Model file for the job. Use its own axes, mm. A direction names the side the tool comes from. Round coordinates to 2 decimals unless told otherwise and drop trailing zeros. Order: outer loops, then holes, each group sorted by start corner. A loop starts at its lowest first (then second) coordinate and runs counter-clockwise, first axis right, second up. Notation, with made-up numbers: M -26,82.25 L 29,82.25 A23 ccw 29,116.25 Z; hole C 2,-23 d1. An arc over 180 degrees is marked long. Return JSON: item names as keys, results as strings. Group by question number.
Item 1: Pull direction Y, two halves, no side cores. Call faces 1 (the face through (129.029, 30.837, 0.74)), 2 (the face through (97, 36.65, 0.74)), 3 (the face through (130.937, 33.329, 0.74)): pulls with the +Y half, pulls with the -Y half, needs draft (parallel to the pull), parting line crosses it, or undercut.
Item 2: Probe line 1 along X through (y, z) = (44, 1.1); line 2 along Y through (x, z) = (36.5, 1.15); line 3 along Y through (x, z) = (79.5, 0.75). List the from-to ranges inside material, lowest first.
Item 3: Slice it at A-A on z = 0.25. Write the cut outline in (x, y).
Item 4: Slice it at B-B on y = 9. Write the cut outline in (x, z), then the cut area to 3 significant figures.
Item 5: Which spindle directions (+Z, -Z, +X, -X, +Y, -Y) get a long thin tool onto all of the face, cutting with end or side? Do faces 4 (the face through (36.141, 48.303, 0.74)), 5 (the face through (11.58, 53.26, 0.76)). Say none if no direction does.
Item 6: Slice it at C-C on x = 32. Write the cut outline in (y, z).
Autodesk Inventor part; units mm, degrees
ref_plane "YZ Plane" through (0, 0, 0) normal (1, 0, 0) x (0, 1, 0)
ref_plane "XZ Plane" through (0, 0, 0) normal (0, 1, 0) x (-1, 0, 0)
ref_plane "XY Plane" through (0, 0, 0) normal (0, 0, 1) x (1, 0, 0)
sketch "スケッチ1" plane through (0, 0, 0) normal (0, 0, 1) x (1, 0, 0)
  circle A0 centre (-35.9404, 22.842) radius 1.5
  circle A1 centre (5.9362, 53.5882) radius 1.5
  circle A2 centre (127.6431, 30.2622) radius 1.5
  line L0 (22.9895, 50.3198) -> (110.5899, 33.5306)
  circle A3 centre (5.9362, 53.5882) radius 4.5
  circle A4 centre (127.6431, 30.2622) radius 4.5
  circle A5 centre (-35.9404, 22.842) radius 3
  line L1 (5.0892, 49.1686) -> (9.9998, 48.2275)
  line L2 (9.9998, 48.2275) -> (22.9895, 50.3198)
  line L3 (110.5899, 33.5306) -> (121.8855, 26.7838)
  line L4 (121.8855, 26.7838) -> (126.7961, 25.8426)
  line L5 (4.4419, 57.8328) -> (15.2047, 61.622)
  line L6 (-37.785, 25.2079) -> (3.1694, 57.1371)
  line L7 (3.5126, 49.7966) -> (-34.0959, 20.4761)
  line L8 (122.0018, 41.1536) -> (130.601, 33.6535)
  circle A6 centre (80.3181, 36.2778) radius 3
  circle A7 centre (80.3181, 36.2778) radius 4.5
  line L9 (128.2106, 34.7263) -> (80.8855, 40.7419)
  circle A8 centre (80.4743, 23.124) radius 1.5
  line L10 (120.4636, 35.711) -> (121.0283, 38.6574)
  line L11 (15.1864, 58.9428) -> (14.6217, 55.9964)
  circle A9 centre (66.9779, 42.9073) radius 1.5
  circle A10 centre (66.9779, 42.9073) radius 3
  line L12 (29.9182, 56.1193) -> (29.3535, 53.1729)
  arc A11 (17.2488, 58.5475) -> (15.1864, 58.9428) centre (16.2176, 58.7451) ccw
  arc A12 (29.9182, 56.1193) -> (27.8558, 56.5146) centre (28.887, 56.3169) ccw
  arc A13 (27.2911, 53.5682) -> (29.3535, 53.1729) centre (28.3223, 53.3705) ccw
  arc A14 (14.6217, 55.9964) -> (16.6841, 55.6011) centre (15.6529, 55.7987) ccw
  line L13 (17.2488, 58.5475) -> (27.8558, 56.5146)
  line L14 (16.6841, 55.6011) -> (27.2911, 53.5682)
  arc A15 (31.8825, 55.7428) -> (27.0019, 58.7146) centre (28.887, 56.3169) ccw
  line L15 (27.0019, 58.7146) -> (18.8556, 60.2759)
  arc A16 (18.8556, 60.2759) -> (15.2047, 61.622) centre (16.2176, 58.7451) ccw
  line L16 (106.2964, 41.4808) -> (105.7317, 38.5345)
  arc A17 (108.3589, 41.0856) -> (106.2964, 41.4808) centre (107.3276, 41.2832) ccw
  arc A18 (121.0283, 38.6574) -> (118.9658, 39.0527) centre (119.997, 38.855) ccw
  arc A19 (118.4011, 36.1063) -> (120.4636, 35.711) centre (119.4323, 35.9086) ccw
  arc A20 (105.7317, 38.5345) -> (107.7942, 38.1392) centre (106.7629, 38.3368) ccw
  line L17 (31.8825, 55.7428) -> (104.3322, 41.8573)
  line L18 (108.3589, 41.0856) -> (118.9658, 39.0527)
  line L19 (107.7942, 38.1392) -> (118.4011, 36.1063)
  arc A21 (122.0018, 41.1536) -> (118.1119, 41.2527) centre (119.997, 38.855) ccw
  line L20 (118.1119, 41.2527) -> (109.9656, 42.814)
  arc A22 (109.9656, 42.814) -> (104.3322, 41.8573) centre (107.3276, 41.2832) ccw
  line L21 (30.451, 58.9354) -> (37.6452, 54.6383)
  line L22 (16.7917, 61.7406) -> (29.4611, 59.3124)
  line L23 (120.5711, 41.8505) -> (107.9017, 44.2787)
  line L24 (106.8426, 44.2944) -> (98.5694, 42.9618)
  point P0 (0, 0)
  point P1 (0, 0)
  dimension "d4" = 9
  dimension "d0" = 9
  dimension "d1" = 9
  dimension "d2" = 6
  dimension "d3" = 6
  dimension "d5" = 47.7059
  dimension "d6" = 47.7059
  dimension "d7" = 3
  dimension "d8" = 3
  dimension "d9" = 8.0769
  dimension "d10" = 8.0769
  dimension "d11" = 3
  dimension "d12" = 6
  dimension "d13" = 61.9691
  dimension "d14" = 61.9691
  dimension "d15" = 15
  dimension "d16" = 2.1
  dimension "d17" = 2
  dimension "d18" = 2
  dimension "d19" = 2
  dimension "d20" = 15
  dimension "d21" = 2.1
  dimension "d22" = 7
  dimension "d23" = 2
  dimension "d24" = 2
  dimension "d25" = 5
  dimension "d26" = 5
  dimension "d27" = 160
  dimension "d28" = 160
  dimension "d29" = 160
  dimension "d30" = 160
sketch "スケッチ2" plane through (0, 0, 0) normal (0, 0, 1) x (1, 0, 0)
  circle A0 centre (5.9362, 53.5882) radius 1.5
  circle A1 centre (66.9779, 42.9073) radius 1.5
  circle A2 centre (127.6431, 30.2622) radius 1.5
  arc A3 (10.3689, 52.8126) -> (1.6172, 52.3248) centre (5.9362, 53.5882) ccw
  arc A4 (71.3832, 41.9891) -> (62.5453, 43.6829) centre (66.9779, 42.9073) ccw
  arc A5 (130.338, 26.6583) -> (123.2378, 31.1804) centre (127.6431, 30.2622) ccw
  line L0 (10.3689, 52.8126) -> (62.5453, 43.6829)
  line L1 (71.3832, 41.9891) -> (123.2378, 31.1804)
  line L2 (130.338, 26.6583) -> (72.4655, -16.6159)
  line L3 (72.4655, -16.6159) -> (15.6298, 4.4202)
  line L4 (15.6298, 4.4202) -> (1.6172, 52.3248)
  point P0 (0, 0)
  dimension "d31" = 9
  dimension "d32" = 9
  dimension "d33" = 9
extrude "押し出し1" add sketch "スケッチ2" along normal blind 1.5
fillet "フィレット1" radius 5 4 edges at (10.3689, 52.8126, 0.75) (62.5453, 43.6829, 0.75) (71.3832, 41.9891, 0.75) (123.2378, 31.1804, 0.75)
equation "\"d6\" = d5"
equation "\"d10\" = d9"
equation "\"d14\" = d13"
properties part number "台形サスカバー" material "ポリカーボネート、クリア"
Output values:
{
 "1": {"face 1": "undercut", "face 2": "pulls with the +Y half", "face 3": "parting line crosses it"},
 "2": {"line 1": "4.05 to 65.95, 68.01 to 71.39", "line 2": "-3.3 to 48.24", "line 3": "-11.36 to 40.3"},
 "3": {"outline": "M 1.62,52.32 L 15.63,4.42 L 72.47,-16.62 L 130.34,26.66 A4.5 ccw long 124.38,33.36 A5 cw 119.74,31.91 L 74.89,41.26 A5 cw 71.21,44.45 A4.5 ccw 63.62,45.9 A5 cw 59.02,44.3 L 13.89,52.2 A5 cw 10.11,55.26 A4.5 ccw Z; hole C 5.94,53.59 d3; hole C 66.98,42.91 d3; hole C 127.64,30.26 d3"},
 "4": {"outline": "M 14.29,0 L 106.72,0 L 106.72,1.5 L 14.29,1.5 Z", "area": "139 mm²"},
 "5": {"face 4": "+Z, -Z, +Y", "face 5": "+Z, -Z, +X, +Y"},
 "6": {"outline": "M -1.64,0 L 49.03,0 L 49.03,1.5 L -1.64,1.5 Z"}
}
